Drawing for the job (mm, zero at the part's lowest x, y, z). A direction names the side the tool comes from. Coordinates: 2 decimals unless noted, no trailing zeros. Write each loop counter-clockwise with the first axis right and the second up, starting at its lowest first coordinate (ties: lowest second). Pieces come first, ordered by that corner, then holes. Notation, with made-up numbers: (56.5, 50.5) -> (79.5, 50.5) arc R22 ccw to (79.5, 73.5) -> close; hole circle Ø7 at (-31.5, 4.25). An arc over 180 degrees is marked (long way). Write each question's results on one line, items separated by ' | '. Start each with the question number.
Q1. Two-plate mould, pull along X, no slides. Class the marked faces 4, 5 and 6: released by +X, released by -X, zero draft, split by the parting line, or undercut.
Q2. Saw through at B-B on z = 5. Give the cut face in (x, y), and give its area (3 significant figures).
Q3. Saw through at A-A on x = 70. Give the cut face in (y, z).
Q4. Drop flat-ended pins along their axis: pin 1 Ø16 at (x, z) = (133.5, 21) entering from -Y; pin 2 Ø1.5 at (x, y) = (86, 16) entering from -Z; pin 3 Ø3 at (y, z) = (23.5, 23.5) entering from +X; pin 4 Ø1.5 at (x, z) = (92, 25.5) entering from -Y. Give the stop position or say it passes through.
Q5. Drill centre lines: line 1 (Y direction, x = 70, z = 16); line 2 (X direction, y = 34, z = 24.25); line 3 (Y direction, x = 11, z = 27). Where is each one in solid material? Low to high.
Q6. Tool access for the marked faces 1, 2 and 3: list every direction of +Z, -Z, +X, -X, +Y, -Y with a clear straight run to the whole face (end or side of a thin tool).
Q7. Saw through at C-C on y = 74. Give the cut face in (x, z), and give its area (3 significant figures).
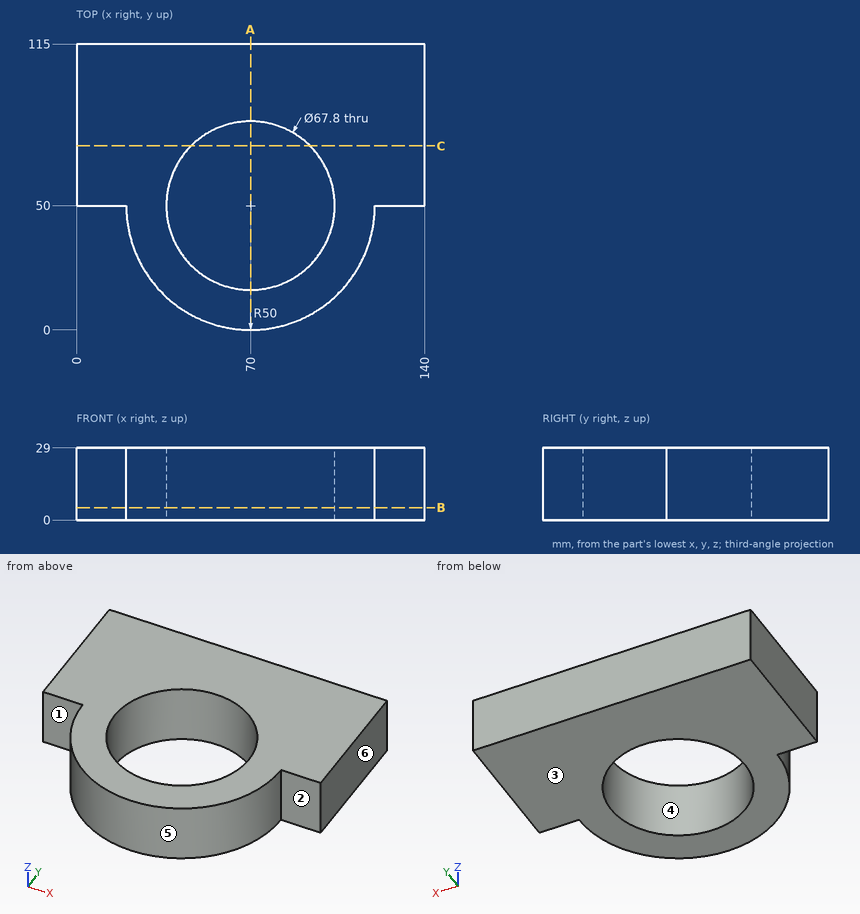
Returned:
1) face 4: undercut | face 5: split by the parting line | face 6: released by +X
2) outline: (0, 50) -> (20, 50) arc R50 ccw to (120, 50) -> (140, 50) -> (140, 115) -> (0, 115) -> close; hole circle Ø67.8 at (70, 50) | area: 9,420 mm2
3) outline: (0, 0) -> (16.1, 0) -> (16.1, 29) -> (0, 29) -> close; (83.9, 0) -> (115, 0) -> (115, 29) -> (83.9, 29) -> close
4) pin 1: stops at y = 50 | pin 2: stops at z = 0 | pin 3: stops at x = 113.3 | pin 4: stops at y = 4.74
5) line 1: y = 0 to 16.1, 83.9 to 115 | line 2: x = 22.63 to 40.11, 99.89 to 117.37 | line 3: y = 50 to 115
6) face 1: +Z, -Z, -X, -Y | face 2: +Z, -Z, +X, -Y | face 3: -Z, +X, -X, +Y, -Y
7) outline: (0, 0) -> (46.06, 0) -> (46.06, 29) -> (0, 29) -> close; (93.94, 0) -> (140, 0) -> (140, 29) -> (93.94, 29) -> close | area: 2,670 mm2
